Design review of the part built by this model. Coordinates are the model's own, in mm. Coordinates: 2 decimals unless noted, no trailing zeros. Order: outer loops, then holes, each group sorted by start corner. A loop starts at its lowest first (then second) coordinate and runs counter-clockwise, first axis right, second up. Notation, with made-up numbers: (59, 68) -> (102, 68) arc R20 ccw to (102, 79) -> close; hole circle Ø10 at (48.25, 16). An arc over 180 degrees is marked (long way). Use a Markdown table: item, result. Add a question column.
Q1. Add section A-A (y = 8). State the section outline as (x, z) points (3 decimals), then the cut area to 3 significant figures.
Q2. Add section C-C (x = 4.2). State the section outline as (y, z) points, then the cut area to 3 significant figures.
Q3. Add section D-D (y = 52.5). State the section outline as (x, z) points (3 decimals).
Q4. Wall thickness on probe 1 along X at (y, z) = (-27.5, 39) (3 decimals); probe 2 along Z at (x, y) = (1.9, 24); probe 3 along Z at (x, y) = (2.15, 46): over which ranges is each line inside the solid? List them lowest first.
Q5. Insertion check: pin 1 (1 mm diameter, centred on x = 2.5, z = 45.5, fed in from +Y); pin 2 (3 mm diameter, centred on x = 4, z = 60.5, fed in from +Y); pin 3 (1.5 mm diameter, centred on x = 1.5, z = 55, fed in from +Y). Each pin has a flat end and moves straight along its axis. Give the tip position at first contact, or say it passes through.
Q6. Add section B-B (z = 41). State the section outline as (x, y) points (3 decimals).
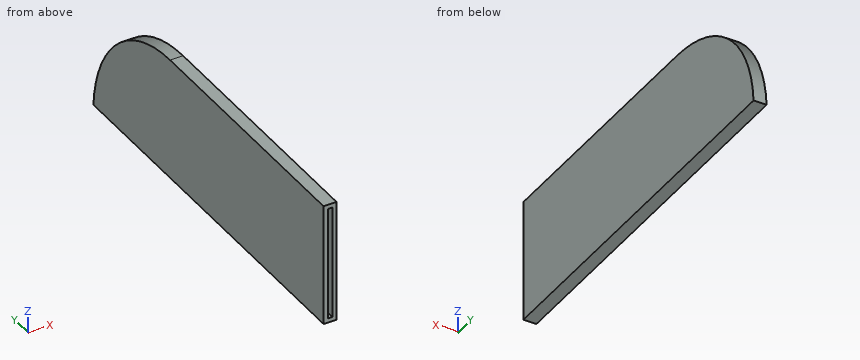
from build123d import *

# Parameters (mm, degrees)
F0_W        = 150
F0_H        = 47
F1_DEPTH    = 5
F2_T1_DEPTH = 254.5495942694
F3_T        = -1.625


# Not quite as in the source:
# - a fillet or chamfer that OpenCascade refuses, or shapes differently, is made with other operations: its cross-section is extruded or revolved along the edge and cut away or added


with BuildPart() as f1:
    # F0 (on Right) → F1 (new body)
    with BuildSketch(Plane.YZ):
        with Locations((9.6287353195, 42.6455706358)):
            Rectangle(F0_W, F0_H)
    extrude(amount=F1_DEPTH)

    # F2: fillet of radius 50 on 1 edges, made by hand

    # F2_s2 → F2_t1 (cut)
    with BuildSketch(Plane.YZ.offset(-124.7747971347)):
        with BuildLine():
            ThreePointArc((84.6287353195, 19.1455706358), (68.9970894677, 52.5461200822), (34.7188164657, 66.1455706358))
            Line((34.7188164657, 66.1455706358), (84.6287353195, 66.1455706358))
            Line((84.6287353195, 66.1455706358), (84.6287353195, 19.1455706358))
        make_face()
    extrude(amount=F2_T1_DEPTH, mode=Mode.SUBTRACT)

    # F3
    f3_openings = [f1.faces().sort_by_distance(p)[0] for p in [
        (2.5, -65.371265, 42.645571),
    ]]
    offset(amount=F3_T, openings=f3_openings)


solid = f1.part
Established:
| question | item | result |
|---|---|---|
| 1 | outline | (0, 19.146) -> (5, 19.146) -> (5, 66.146) -> (0, 66.146) -> close; hole (1.625, 20.771) -> (3.375, 20.771) -> (3.375, 64.521) -> (1.625, 64.521) -> close |
| 1 | area | 158 mm^2 |
| 2 | outline | (-65.37, 19.15) -> (84.63, 19.15) arc R50 ccw to (34.72, 66.15) -> (-65.37, 66.15) -> close |
| 2 | area | 6,520 mm^2 |
| 3 | outline | (0, 19.146) -> (5, 19.146) -> (5, 62.877) -> (0, 62.877) -> close; hole (1.625, 20.771) -> (3.375, 20.771) -> (3.375, 61.134) -> (1.625, 61.134) -> close |
| 4 | probe 1 | 0 to 1.625, 3.375 to 5 |
| 4 | probe 2 | 19.15 to 20.77, 64.52 to 66.15 |
| 4 | probe 3 | 19.15 to 20.77, 63.19 to 64.86 |
| 5 | pin 1 | y = 75.55 |
| 5 | pin 2 | y = 60.48 |
| 5 | pin 3 | y = 67.09 |
| 6 | outline | (0, -65.371) -> (1.625, -65.371) -> (1.625, 76.221) -> (3.375, 76.221) -> (3.375, -65.371) -> (5, -65.371) -> (5, 78.104) -> (0, 78.104) -> close |
